Design review of the part built by this model. Coordinates are the model's own, in mm. A direction names the side the tool comes from. Round coordinates to 2 decimals unless told otherwise and drop trailing zeros. Order: outer loops, then holes, each group sorted by start corner. A loop starts at its lowest first (then second) coordinate and runs counter-clockwise, first axis right, second up.
from build123d import *

# Parameters (mm, degrees)
SKETCH1_W            = 7.5
SKETCH1_H            = 7
SKETCH2_W            = 3
SKETCH2_H            = 5
SKETCH2_W_2          = 5
SKETCH2_H_2          = 3
CUT_4XSLOT_5X2_DEPTH = 150


with BuildPart() as part:
    # Sketch1 → REV_KM6_M30x1.5_45x7 (revolve)
    with BuildSketch(Plane(origin=(0, 0, 0), x_dir=(1, 0, 0), z_dir=(0, 1, 0))):
        with Locations((18.75, 92.5)):
            Rectangle(SKETCH1_W, SKETCH1_H)
    revolve(axis=Axis((0, 0, 150), (0, 0, -1)))

    # Sketch2 → CUT_4xSlot_5x2 (cut, symmetric)
    with BuildSketch(Plane.XY):
        with Locations((22, 0)):
            Rectangle(SKETCH2_W, SKETCH2_H)
        with Locations((-22, 0)):
            Rectangle(SKETCH2_W, SKETCH2_H)
        with Locations((0, 22)):
            Rectangle(SKETCH2_W_2, SKETCH2_H_2)
        with Locations((0, -22)):
            Rectangle(SKETCH2_W_2, SKETCH2_H_2)
    extrude(amount=CUT_4XSLOT_5X2_DEPTH, both=True, mode=Mode.SUBTRACT)


solid = part.part
1) Take a section at C-C on z = -94.5. Give the boundary of the cut face in (x, y).
Results:
outline: (-22.36, -2.5) arc R22.5 ccw to (-2.5, -22.36) - (-2.5, -20.5) - (2.5, -20.5) - (2.5, -22.36) arc R22.5 ccw to (22.36, -2.5) - (20.5, -2.5) - (20.5, 2.5) - (22.36, 2.5) arc R22.5 ccw to (2.5, 22.36) - (2.5, 20.5) - (-2.5, 20.5) - (-2.5, 22.36) arc R22.5 ccw to (-22.36, 2.5) - (-20.5, 2.5) - (-20.5, -2.5) - close; hole circle Ø30 at (0, 0)
2) Take a section at A-A on y = 0. Give the boundary of the cut face in (x, z), plus the area to 3 significant figures.
Results:
outline: (-20.5, -96) - (-15, -96) - (-15, -89) - (-20.5, -89) - close; (15, -96) - (20.5, -96) - (20.5, -89) - (15, -89) - close
area: 77.0 mm2
3) To check wall thickness, follow line 1 along Y through (x, z) = (0, -92.5); line 2 along Y through (x, z) = (-13, -91.5). State the ranges of each line that lie inside material, in increasing order.
Results:
line 1: y = -20.5 to -15, 15 to 20.5
line 2: y = -18.36 to -7.48, 7.48 to 18.36
4) Take a section at D-D on y = 18. Give the boundary of the cut face in (x, z), plus the area to 3 significant figures.
Results:
outline: (-13.5, -96) - (13.5, -96) - (13.5, -89) - (-13.5, -89) - close
area: 189 mm2
5) For faces 1 (the face through (-2.5, -21, -92)), 2 (the face through (21, 2.5, -93)), 3 (the face through (-20.5, 0, -93)), 4 (the face through (2.5, 21, -93)), list the 3-axis set-ups (+Z, -Z, +X, -X, +Y, -Y) from which the entire face can be reached by the end or side of a thin tool; tool diameter is ignored.
Results:
face 1: +Z, -Z, -Y
face 2: +Z, -Z, +X
face 3: +Z, -Z, -X
face 4: +Z, -Z, +Y
6) The part is to be moulded in two halves that separate along Y. For faces 5 (the face through (0, 20.5, -93)), 6 (the face through (-21, -2.5, -93)), 7 (the face through (0, -20.5, -92)), 8 (the face through (-21, 2.5, -93)), say which applies: released by +Y, released by -Y, zero draft, split by the parting line, or undercut.
Results:
face 5: released by +Y
face 6: undercut
face 7: released by -Y
face 8: undercut
7) Clearance check with flat-ended pins moving along their axes: P1, Ø2, axis at y = 21, z = -92, coming from the +X side; P2, Ø3, axis at x = 1.5, y = -14, coming from the +Z side; P3, Ø0.6, axis at y = -21, z = -92.5, coming from the +X side; P4, Ø4, axis at y = 8.5, z = -92.5, coming from the +X side. State where each tip first meets the part, or that it passes through.
Results:
P1: stops at x = 10.31
P2: stops at z = -89
P3: stops at x = 8.82
P4: stops at x = 21.54
